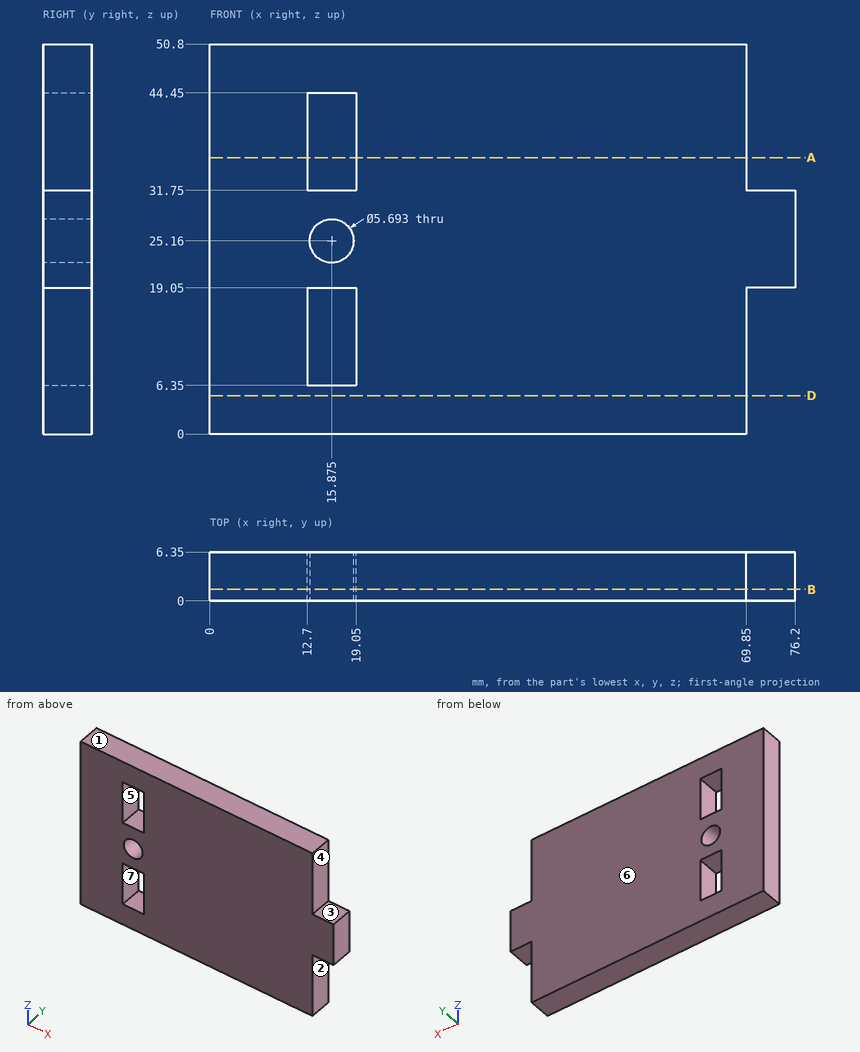
Verification items for this drawing (mm, ordinates from the low corner). A direction names the side the tool comes from. Give positions to 0.01 mm unless a question says otherwise; leave off trailing zeros. Write each loop counter-clockwise with the first axis right and the second up, starting at its lowest first coordinate (ties: lowest second). Pieces come first, ordered by that corner, then holes. Notation, with made-up numbers: (54.25, -27) -> (96.25, -27) arc R3 cw to (96.25, -23) -> close; hole circle Ø7 at (69, 70). An arc over 180 degrees is marked (long way). Use CSV: the item, a comma, the result in double quotes. Start each with the question number.
Q1. Release check for a two-part mould opening along X. For the marked faces 4, 5, 6 and 7 record: +X half, -X half, draft (parallel to the pull), parting line (faces both ways), or undercut.
Q2. Cross-section at A-A on z = 36. Enter the section's corners in (x, y).
Q3. Scan lines: line 1 along X through (y, z) = (5, 42.5); line 2 along Z through (x, y) = (14.5, 2.5); line 3 along X through (y, z) = (1, 5). Record each from-to range of solid material in increasing order.
Q4. Cross-section at D-D on z = 5. Enter the section's corners in (x, y).
Q5. Cross-section at B-B on y = 1.5. Count the separate pieces of the cut face and the enclosed holes in it, and give its area (3 significant figures).
Q6. Tool access check on the marked faces 1, 2 and 3. Record the directions out of +Z, -Z, +X, -X, +Y, -Y that give a thin tool (end or side, any length) a straight path to the whole face; none if there is none.
Q7. Depth check by flat-ended pin: P1, Ø3, axis at x = 71.5, y = 4, coming from the +Z side; P2, Ø1.9, axis at y = 4, z = 37.5, coming from the +X side. Enter the tip coordinate at first touch or a pass-through.
Working result:
1,face 4,"+X half"
1,face 5,"undercut"
1,face 6,"draft"
1,face 7,"undercut"
2,outline,"(0, 0) -> (12.7, 0) -> (12.7, 6.35) -> (0, 6.35) -> close; (19.05, 0) -> (69.85, 0) -> (69.85, 6.35) -> (19.05, 6.35) -> close"
3,line 1,"x = 0 to 12.7, 19.05 to 69.85"
3,line 2,"z = 0 to 6.35, 19.05 to 22.67, 27.65 to 31.75, 44.45 to 50.8"
3,line 3,"x = 0 to 69.85"
4,outline,"(0, 0) -> (69.85, 0) -> (69.85, 6.35) -> (0, 6.35) -> close"
5,separate pieces,"1"
5,enclosed holes,"3"
5,area,"3,440 mm^2"
6,face 1,"+Z, +X, -X, +Y, -Y"
6,face 2,"-Z, +X, +Y, -Y"
6,face 3,"+Z, +X, +Y, -Y"
7,P1,"stops at z = 31.75"
7,P2,"stops at x = 69.85"
